Check sheet for the modelled part. Datum: model origin and axes. Units: mm. A direction names the side the tool comes from. Give positions to 0.01 mm unless a question says otherwise; leave off trailing zeros. Loops run counter-clockwise (first coordinate to the right, second up) from the corner with the lowest first, then second, coordinate; pieces in that order, holes last. Notation, with made-up numbers: M 7.5,10 L 50.5,10 A9 ccw 50.5,16 Z; hole C 58,-32 d10. An arc over 180 degrees is marked long. Write each question's results on one line, items separated by ' | '. Start each with the question number.
1. Sectioned sample at B-B on z = -23. Record the cut outline in (x, y) (3 decimals).
2. Draft check along Y on faces 4 (the flat face through (-89, 0, 0)), 5 (the flat face through (76, -31.75, -5)), 6 (the cylindrical face through (-109.976, 23.636, -4.696)). Enter one of: pulls with the +Y half, pulls with the -Y half, needs draft (parallel to the pull), parting line crosses it, or undercut.
3. Tool access check on faces 1 (the flat face through (-6, -9.525, -75)), 2 (the flat face through (44.426, 0, -5)), 3 (the flat face through (69, 0, -9.525)). Record the directions out of +Z, -Z, +X, -X, +Y, -Y that give a thin tool (end or side, any length) a straight path to the whole face; none if there is none.
4. Sectioned sample at C-C on x = 86. Record the cut outline in (y, z) (3 decimals).
5. Go/stop test with flat-tipped pins: pin 1 (12 mm diameter, centred on x = -80, z = -42.5, fed in from -Y) (3 decimals); pin 2 (3.5 mm diameter, centred on x = -112.64, y = 22.8, fed in from +Z); pin 3 (19 mm diameter, centred on x = 74, y = 11.5, fed in from -Z); pin 4 (8 mm diameter, centred on x = 47, y = -14, fed in from -Z) (3 decimals). Record where each tip stops, or that it passes through.
6. Sectioned sample at A-A on y = -12. Record the cut outline in (x, z) (3 decimals), and give its area (3 significant figures).
7. Sectioned sample at D-D on z = -80. Record the cut outline in (x, y) (3 decimals).
8. Material ranges on line 1 along X through (y, z) = (-6.5, -9); line 2 along Y through (x, z) = (45, -76.5) (3 decimals); line 3 along Z through (x, y) = (-67, -20) (3 decimals), recorded low to high.
```python
from build123d import *

# Parameters (mm, degrees)
F1_W     = 19.05
F1_H     = 19.05
F2_ANGLE = 180
F0_W     = 63.5
F0_H     = 63.5
F0_R     = 2.794
F3_DEPTH = 9.525
F4_DEPTH = 9.525


with BuildPart() as f2:
    # F1 (on Top) → F2 (revolve)
    with BuildSketch(Plane.XY):
        with Locations((-82.55, 0)):
            Rectangle(F1_W, F1_H)
    revolve(axis=Axis((0, 0, 0), (0, -1, 0)), revolution_arc=F2_ANGLE)

    # F0 (on Top) → F3 (join)
    with BuildSketch(Plane.XY):
        with Locations((-88.923662, 0)):
            Rectangle(F0_W, F0_H)
        with Locations((-112.640873, 22.796268)):
            Circle(F0_R, mode=Mode.SUBTRACT)
    extrude(amount=-F3_DEPTH)

    # F0 (on Top) + F1 (on Top) → F4 (join)
    with BuildSketch(Plane.XY):
        with Locations((76.176338, 0)):
            Rectangle(F0_W, F0_H)
    with BuildSketch(Plane.XY):
        with Locations((-82.55, 0)):
            Rectangle(F1_W, F1_H)
    extrude(amount=-F4_DEPTH)


solid = f2.part
```
Output values:
1) outline: M -89.156,-9.525 L -69.308,-9.525 L -69.308,9.525 L -89.156,9.525 Z; M 69.308,-9.525 L 89.156,-9.525 L 89.156,9.525 L 69.308,9.525 Z
2) face 4: needs draft | face 5: pulls with the -Y half | face 6: undercut
3) face 1: -Z, +X, -X, -Y | face 2: +Z, +Y, -Y | face 3: none
4) outline: M -31.75,-9.525 L -9.525,-9.525 L -9.525,-32.891 L 9.525,-32.891 L 9.525,-9.525 L 31.75,-9.525 L 31.75,0 L -31.75,0 Z
5) pin 1: y = -9.525 | pin 2: through | pin 3: z = -65.5 | pin 4: z = -9.525
6) outline: M -120.674,-9.525 L -57.174,-9.525 L -57.174,0 L -120.674,0 Z; M 44.426,-9.525 L 107.926,-9.525 L 107.926,0 L 44.426,0 Z | area: 1,210 mm2
7) outline: M -45.583,-9.525 L 45.583,-9.525 L 45.583,9.525 L -45.583,9.525 Z
8) line 1: -120.67 to -57.17, 44.43 to 107.93 | line 2: -9.525 to 9.525 | line 3: -9.525 to 0
